Check sheet for the modelled part. Datum: model origin and axes. Units: mm. Face numbers are marked on the shaded views. A direction names the side the tool comes from. Coordinates: 2 decimals unless noted, no trailing zeros. Loops run counter-clockwise (first coordinate to the right, second up) from the corner with the lowest first, then second, coordinate; pieces in that order, holes last. Notation, with made-up numbers: M 22.25,66.5 L 69.25,66.5 A15 ccw 69.25,90.5 Z; hole C 1.5,-39.75 d6. An arc over 180 degrees is marked long. Return JSON: item names as keys, results as strings.
from build123d import *

# Parameters (mm, degrees)
F1_DEPTH = 60.198
F0_W     = 10.922
F0_H     = 16.735694
F0_H_2   = 27.714306
F2_DEPTH = 50.8
F3_DEPTH = 10.922
F4_R     = 6.642507
F5_DEPTH = 10.923
F6_SIZE2 = 16.571107
F6_SIZE  = 28.702
F7_SIZE2 = 22.119206
F7_SIZE  = 82.55


with BuildPart() as f1:
    # F0 (on Top) → F1 (new body)
    with BuildSketch(Plane.XY):
        Polygon((-8.589479, 19.945886), (-40.339479, 19.945886), (-40.339479, 9.023886), (-29.417479, 9.023886), (-8.589479, 9.023886), align=None)
        Polygon((73.960521, 19.945886), (-8.589479, 19.945886), (-8.589479, 9.023886), (29.338112, 9.023886), (73.960521, 9.023886), align=None)
    extrude(amount=F1_DEPTH)

    # F0 (on Top) → F2 (join)
    with BuildSketch(Plane.XY):
        with Locations((-34.878479, 0.656039)):
            Rectangle(F0_W, F0_H)
        with Locations((-34.878479, -21.568961)):
            Rectangle(F0_W, F0_H_2)
    extrude(amount=F2_DEPTH)

    # F0 (on Top) → F3 (join)
    with BuildSketch(Plane.XY):
        Polygon((29.338112, 9.023886), (-8.589479, 9.023886), (-29.417479, 9.023886), (-29.417479, -7.711808), (-29.417479, -35.426114), align=None)
    extrude(amount=F3_DEPTH)

    # F4 (on face) → F5 (cut, through all)
    with BuildSketch(Plane.XZ.offset(-9.023886)):
        with Locations((54.910521, 19.05)):
            Circle(F4_R)
    extrude(amount=-F5_DEPTH, mode=Mode.SUBTRACT)

    # F6
    f6_edges = [f1.edges().sort_by_distance(p)[0] for p in [
        (-34.878479, -35.426114, 50.8),
    ]]
    chamfer(f6_edges, length=F6_SIZE, length2=F6_SIZE2)

    # F7
    f7_edges = [f1.edges().sort_by_distance(p)[0] for p in [
        (73.960521, 14.484886, 60.198),
    ]]
    chamfer(f7_edges, length=F7_SIZE, length2=F7_SIZE2)


solid = f1.part
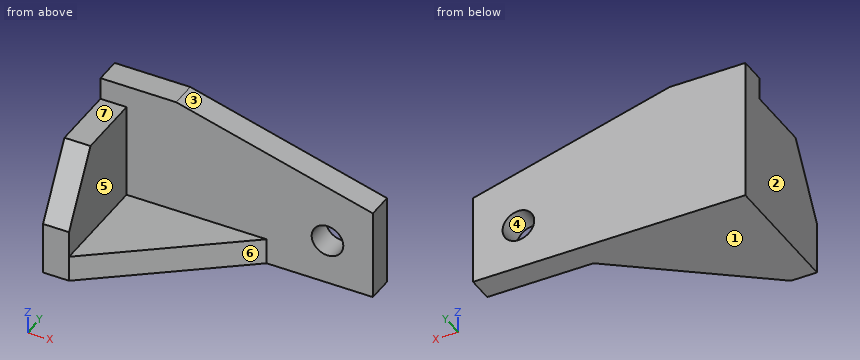
1) Section check C-C on z = 5. Record the cut outline in (x, y).
Answers:
{"outline": "M -40.34,-35.43 L -29.42,-35.43 L 29.34,9.02 L 73.96,9.02 L 73.96,19.95 L -40.34,19.95 Z"}
2) Scan lines: line 1 along X through (y, z) = (8.5, 46.5); line 2 along Z through (x, y) = (-25.5, -31.5); line 3 along Y through (x, z) = (6, 52.5). Record each from-to range of solid material in increasing order. Write a range as [from, to].
Answers:
{"line 1": "[-40.34, -29.42]", "line 2": "[0, 10.92]", "line 3": "[9.02, 19.95]"}
3) Section check D-D on x = -1.5. Record the cut outline in (y, z), then the cut area to 3 significant figures.
Answers:
{"outline": "M -14.31,0 L 19.95,0 L 19.95,58.3 L 9.02,58.3 L 9.02,10.92 L -14.31,10.92 Z", "area": "892 mm²"}
4) Section check A-A on z = 19.05. Record the cut outline in (x, y), then the cut area to 3 significant figures.
Answers:
{"outline": "M -40.34,-35.43 L -29.42,-35.43 L -29.42,9.02 L 48.27,9.02 L 48.27,19.95 L -40.34,19.95 Z; M 61.55,9.02 L 73.96,9.02 L 73.96,19.95 L 61.55,19.95 Z", "area": "1,590 mm²"}
5) Section check B-B on y = 10.5. Record the cut outline in (x, z), then the cut area to 3 significant figures.
Answers:
{"outline": "M -40.34,0 L 73.96,0 L 73.96,38.08 L -8.59,60.2 L -40.34,60.2 Z; hole C 54.91,19.05 d13.29", "area": "5,830 mm²"}
6) Set-up check for the marked faces 5, 6 and 7: record each of +Z, -Z, +X, -X, +Y, -Y from which the full face is reachable in a straight line by a thin tool's end or side.
Answers:
{"face 5": "+Z, +X, -Y", "face 6": "+Z, -Z, +X, -Y", "face 7": "+Z, +X, -X, -Y"}
7) Go/stop test with flat-tipped pins: pin 1 Ø10 at (x, z) = (15, 14) entering from -Y; pin 2 Ø5.5 at (x, y) = (-34.5, 2) entering from +Z; pin 3 Ø6 at (y, z) = (-15, 50.5) entering from +X. Record where each tip stops, or that it passes through.
Answers:
{"pin 1": "y = -4.8", "pin 2": "z = 50.8", "pin 3": "x = -29.42"}
8) Draft check along Z on the marked faces 1, 2, 3 and 4. Enter one of: +Z half, -Z half, draft (parallel to the pull), parting line (faces both ways), or undercut.
Answers:
{"face 1": "-Z half", "face 2": "draft", "face 3": "+Z half", "face 4": "undercut"}
